from build123d import *

# Parameters (mm, degrees)
F0_R     = 9.3218
F1_DEPTH = 1.524
F2_R     = 7.7724
F3_DEPTH = 8.636
F4_R     = 6.35
F5_DEPTH = 10.161


with BuildPart() as f1:
    # F0 (on Top) → F1 (new body)
    with BuildSketch(Plane.XY):
        Circle(F0_R)
    extrude(amount=F1_DEPTH)

    # F2 (on face) → F3 (join)
    with BuildSketch(Plane(origin=(0, 0, 0), x_dir=(1, 0, 0), z_dir=(0, 0, -1))):
        Circle(F2_R)
    extrude(amount=F3_DEPTH)

    # F4 (on face) → F5 (cut, through all)
    with BuildSketch(Plane.XY.offset(1.524)):
        Circle(F4_R)
    extrude(amount=-F5_DEPTH, mode=Mode.SUBTRACT)


solid = f1.part
Can you work these out from the model? Positions are in its coordinate system, mm. A direction names the side the tool comes from. Round coordinates to 2 decimals unless told otherwise and drop trailing zeros. Loops run counter-clockwise (first coordinate to the right, second up) from the corner with the lowest first, then second, coordinate; pieces in that order, holes last. Notation, with made-up numbers: (5, -33) - (47, -33) arc R20 cw to (47, -10) - close; hole circle Ø9 at (82, 42). An arc over 180 degrees is marked (long way). Write item = value, one per line. Start each with the question number.
(1) If we section it at A-A (x = 0): Please give me the cut outline in (y, z).
(2) If I drill on probe 1 along Y at (x, z) = (0, -6.5); probe 2 along Y at (x, z) = (-0.25, 1); probe 3 along Z at (x, y) = (-4.5, 7.25), over which ranges is the centre line in solid material (lowest first)? Write a range as [from, to].
(3) For faces 1 (the face through (8.89, 2.8, 0.75)), 2 (the face through (2, -8, 0)), which set-ups out of +Z, -Z, +X, -X, +Y, -Y let a thin tool reach every point of the face, with its end or its side?
(4) If we section it at D-D (y = 7): Please give me the cut outline in (x, z), and give its area (3 significant figures).
(5) For P1, Ø1, axis at x = 7, z = -5, coming from the -Y side; P2, Ø1, axis at y = -2.5, z = 0, coming from the -X side; P3, Ø1, axis at x = -5, z = -1.5, coming from the -Y side, each with a flat end and sliding along its axis, tell me the tip position at first contact or that it passes through.
(6) If we mould it in two halves opening along Y, with no side actions, what happens to faces 3 (the face through (7.413, -2.335, -4.258)), 4 (the face through (4, -6, 1.524)), 5 (the face through (-1.38, -6.2, -3.48))? For each: released by +Y, released by -Y, zero draft, split by the parting line, or undercut.
(7) If we section it at C-C (z = -3.5): Please give me the cut outline in (x, y).
Ans:
q1.outline = (-9.32, 0) - (-7.77, 0) - (-7.77, -8.64) - (-6.35, -8.64) - (-6.35, 1.52) - (-9.32, 1.52) - close; (6.35, -8.64) - (7.77, -8.64) - (7.77, 0) - (9.32, 0) - (9.32, 1.52) - (6.35, 1.52) - close
q2.probe_1 = [-7.77, -6.35], [6.35, 7.77]
q2.probe_2 = [-9.32, -6.35], [6.35, 9.32]
q2.probe_3 = [0, 1.52]
q3.face_1 = +Z, -Z
q3.face_2 = -Z
q4.outline = (-6.16, 0) - (-3.38, 0) - (-3.38, -8.64) - (3.38, -8.64) - (3.38, 0) - (6.16, 0) - (6.16, 1.52) - (-6.16, 1.52) - close
q4.area = 77.1 mm²
q5.P1 = -4.26
q5.P2 = -9.1
q5.P3 = -6.34
q6.face_3 = split by the parting line
q6.face_4 = zero draft
q6.face_5 = undercut
q7.outline = circle Ø15.54 at (0, 0); hole circle Ø12.7 at (0, 0)
